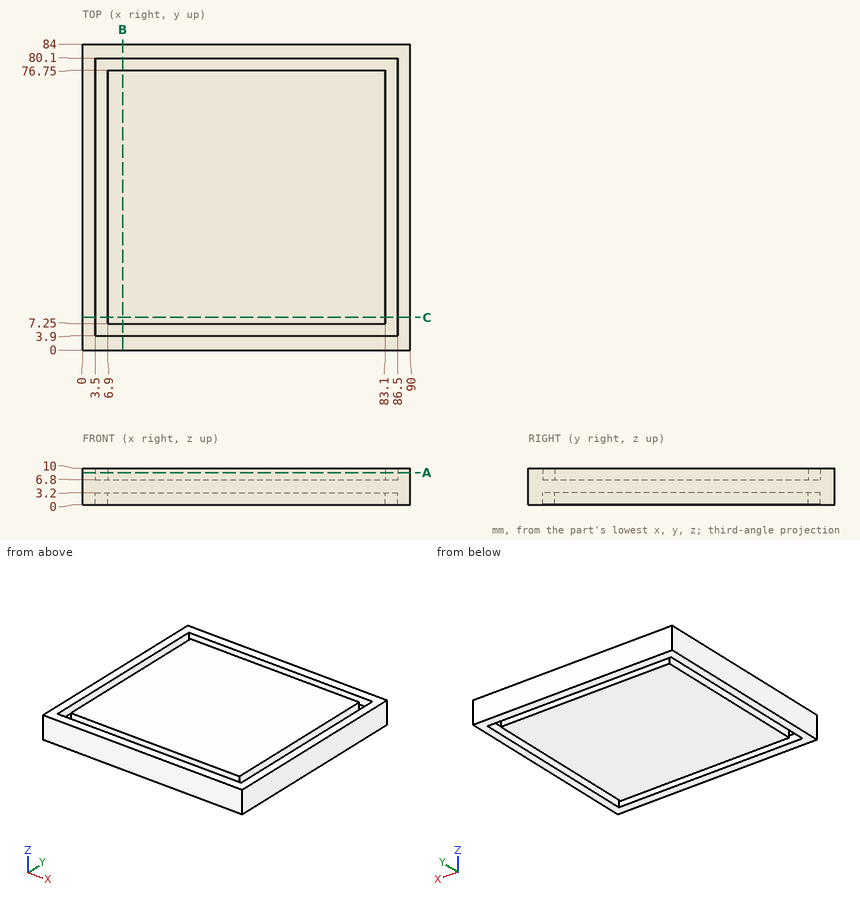
Geometry check sheet. Reference: drawing and pictorial views, mm from the part's lowest x, y, z. Give positions to 0.01 mm unless a question says otherwise; leave off trailing zeros. Order: outer loops, then holes, each group sorted by start corner. A loop starts at its lowest first (then second) coordinate and runs counter-clockwise, first axis right, second up. Notation, with made-up numbers: (81.5, -4.75) -> (135.5, -4.75) arc R21 cw to (135.5, 12.25) -> close; hole circle Ø10 at (39, 25.5). An arc over 180 degrees is marked (long way). Use CSV: the item, a comma, the result in double quotes. Start each with the question number.
1) Sectioned sample at A-A, the plane z = 8.75. Record the boundary of the cut face in (x, y), plus the area to 3 significant figures.
2) Go/stop test with a flat-tipped pin: P1, Ø1.6, axis at y = 32.5, z = 1.5, coming from the -X side. Record where the tip stops, or that it passes through.
3) Sectioned sample at B-B, the plane x = 11. Record the boundary of the cut face in (y, z).
4) Sectioned sample at C-C, the plane y = 9. Record the boundary of the cut face in (x, z).
5) Material ranges on line 1 (Y direction, x = 68, z = 7); line 2 (X direction, y = 52, z = 9.5); line 3 (X direction, y = 6.5, z = 2.25), recorded low to high. Write a range as from..to.
Recorded:
1,outline,"(0, 0) -> (90, 0) -> (90, 84) -> (0, 84) -> close; (6.9, 7.25) -> (83.1, 7.25) -> (83.1, 76.75) -> (6.9, 76.75) -> close; hole (3.5, 3.9) -> (86.5, 3.9) -> (86.5, 80.1) -> (3.5, 80.1) -> close"
1,area,"6,530 mm2"
2,P1,"x = 0"
3,outline,"(0, 0) -> (3.9, 0) -> (3.9, 3.2) -> (7.25, 3.2) -> (7.25, 0) -> (76.75, 0) -> (76.75, 3.2) -> (80.1, 3.2) -> (80.1, 0) -> (84, 0) -> (84, 10) -> (80.1, 10) -> (80.1, 6.8) -> (76.75, 6.8) -> (76.75, 10) -> (7.25, 10) -> (7.25, 6.8) -> (3.9, 6.8) -> (3.9, 10) -> (0, 10) -> close"
4,outline,"(0, 0) -> (3.5, 0) -> (3.5, 3.2) -> (6.9, 3.2) -> (6.9, 0) -> (83.1, 0) -> (83.1, 3.2) -> (86.5, 3.2) -> (86.5, 0) -> (90, 0) -> (90, 10) -> (86.5, 10) -> (86.5, 6.8) -> (83.1, 6.8) -> (83.1, 10) -> (6.9, 10) -> (6.9, 6.8) -> (3.5, 6.8) -> (3.5, 10) -> (0, 10) -> close"
5,line 1,"0..3.9, 7.25..76.75, 80.1..84"
5,line 2,"0..3.5, 6.9..83.1, 86.5..90"
5,line 3,"0..3.5, 86.5..90"
